```python
from build123d import *

# Parameters (mm, degrees)
SKETCH1_W           = 60
SKETCH1_H           = 15
SKETCH1_R           = 1
BOSS_EXTRUDE1_DEPTH = 4
FILLET1_RADIUS      = 7.5
FILLET1_LENGTH      = 4
FILLET2_RADIUS      = 7.5
FILLET2_LENGTH      = 4
CUT_EXTRUDE1_DEPTH  = 2
SKETCH4_R           = 3.5
CUT_EXTRUDE2_DEPTH  = 6
CUT_EXTRUDE3_DEPTH  = 2
SKETCH6_R           = 3.5
CUT_EXTRUDE4_DEPTH  = 6


with BuildPart() as part:
    # Sketch1 → Boss-Extrude1 (new body)
    with BuildSketch(Plane.XY):
        with Locations((-25, 9.186746988)):
            Rectangle(SKETCH1_W, SKETCH1_H)
        with Locations((-50, 9.186746988)):
            Circle(SKETCH1_R, mode=Mode.SUBTRACT)
        with Locations((0, 9.186746988)):
            Circle(SKETCH1_R, mode=Mode.SUBTRACT)
    extrude(amount=BOSS_EXTRUDE1_DEPTH)

    # Fillet1: full round fillet: the end face becomes a half cylinder, R = half its width
    fillet1_face = Plane((5, 9.186746988, 2), x_dir=(0, 0, -1), z_dir=(1, 0, 0))  # on the end face: x along it, z out of the body
    fillet1_slab = fillet1_face.offset(-FILLET1_RADIUS / 2) * Box(FILLET1_LENGTH, 2 * FILLET1_RADIUS, FILLET1_RADIUS, mode=Mode.PRIVATE)  # the body's end, R deep
    fillet1_round = Plane((-2.5, 9.186746988, 2), x_dir=(1, 0, 0), z_dir=(0, 0, -1)) * Cylinder(FILLET1_RADIUS, FILLET1_LENGTH, mode=Mode.PRIVATE)  # its axis R under the face
    add(fillet1_slab - fillet1_round, mode=Mode.SUBTRACT)

    # Fillet2: full round fillet: the end face becomes a half cylinder, R = half its width
    fillet2_face = Plane((-55, 9.186746988, 2), x_dir=(0, 0, 1), z_dir=(-1, 0, 0))  # on the end face: x along it, z out of the body
    fillet2_slab = fillet2_face.offset(-FILLET2_RADIUS / 2) * Box(FILLET2_LENGTH, 2 * FILLET2_RADIUS, FILLET2_RADIUS, mode=Mode.PRIVATE)  # the body's end, R deep
    fillet2_round = Plane((-47.5, 9.186746988, 2), x_dir=(-1, 0, 0), z_dir=(0, 0, 1)) * Cylinder(FILLET2_RADIUS, FILLET2_LENGTH, mode=Mode.PRIVATE)  # its axis R under the face
    add(fillet2_slab - fillet2_round, mode=Mode.SUBTRACT)

    # Sketch3 → Cut-Extrude1 (cut)
    with BuildSketch(Plane(origin=(0, 0, 0), x_dir=(-1, 0, 0), z_dir=(0, 0, -1))):
        with BuildLine():
            Line((14.214285714, 11.17523426), (0.375, 12.666599715))
            ThreePointArc((0.375, 12.666599715), (-3.5, 9.186746988), (0.375, 5.706894261))
            Line((0.375, 5.706894261), (14.214285714, 7.198259716))
            ThreePointArc((14.214285714, 7.198259716), (16, 9.186746988), (14.214285714, 11.17523426))
        make_face()
    extrude(amount=-CUT_EXTRUDE1_DEPTH, mode=Mode.SUBTRACT)

    # Sketch4 → Cut-Extrude2 (cut)
    with BuildSketch(Plane(origin=(0, 0, 2), x_dir=(-1, 0, 0), z_dir=(0, 0, -1))):
        with Locations(Location((0, 9.186746988, 0), (0, 0, 276.150639828))):
            Circle(SKETCH4_R)
    extrude(amount=-CUT_EXTRUDE2_DEPTH, mode=Mode.SUBTRACT)

    # Sketch5 → Cut-Extrude3 (cut)
    with BuildSketch(Plane(origin=(0, 0, 0), x_dir=(-1, 0, 0), z_dir=(0, 0, -1))):
        with BuildLine():
            Line((49.625, 12.666599715), (35.785714286, 11.17523426))
            ThreePointArc((35.785714286, 11.17523426), (34, 9.186746988), (35.785714286, 7.198259716))
            Line((35.785714286, 7.198259716), (49.625, 5.706894261))
            ThreePointArc((49.625, 5.706894261), (53.5, 9.186746988), (49.625, 12.666599715))
        make_face()
    extrude(amount=-CUT_EXTRUDE3_DEPTH, mode=Mode.SUBTRACT)

    # Sketch6 → Cut-Extrude4 (cut)
    with BuildSketch(Plane(origin=(0, 0, 0), x_dir=(-1, 0, 0), z_dir=(0, 0, -1))):
        with Locations(Location((50, 9.186746988, 0), (0, 0, 96.150639828))):
            Circle(SKETCH6_R)
    extrude(amount=-CUT_EXTRUDE4_DEPTH, mode=Mode.SUBTRACT)


solid = part.part
```
Source: CAD feature listing. Evaluate the final solid. Frame: model axes, mm. A direction names the side the tool comes from. Round coordinates to 2 decimals unless told otherwise and drop trailing zeros. Write each loop counter-clockwise with the first axis right and the second up, starting at its lowest first coordinate (ties: lowest second). Pieces come first, ordered by that corner, then holes. Notation, with made-up numbers: M -29.5,1 L -14.5,1 A31 ccw -14.5,32 Z; hole C -38,-37 d7. An arc over 180 degrees is marked long. Answer as a JSON object with one key per item and string values. Group by question number.
(1) Section query C-C on y = 9.25. Output: boundary loops of the cut face in (x, z), then the cut area to 3 significant figures.
(2) Reachability of faces 1 (the flat face through (-25, 9, 4)), 2 (the flat face through (-42.608, 6.463, 0.986)) from +Z, -Z, +X, -X, +Y, -Y: full face, straight path, thin tool, end or side. Return the list, or none.
(3) First-contact query: pin 1 (2 mm diameter, centred on x = -39.5, y = 9, fed in from -Z); pin 2 (7.5 mm diameter, centred on x = -7.5, y = 8.5, fed in from -Z). Flat tips, straight axial feed; report the tip coordinate or a pass-through.
(4) Ray query, line 1 (X direction, y = 11, z = 1.1); line 2 (X direction, y = 6.25, z = 2.4); line 3 (Z direction, x = -41, y = 11.5). Return the intervals inside material, ascending. Write a range as [from, to].
(5) Mould query, pull axis Y, two halves, no side actions, for faces 3 (the flat face through (-7.198, 6.442, 0.986)), 4 (the cylindrical face through (-55, 9.35, 2.03)), 5 (the flat face through (-25, 1.687, 2)). Classes: +Y half, -Y half, draft (parallel to the pull), parting line (faces both ways), or undercut.
(6) Section query D-D on z = 3.05. Output: boundary loops of the cut face in (x, y) (3 decimals), then the cut area to 3 significant figures.
(7) Section query A-A on x = -48.5. Output: boundary loops of the cut face in (y, z).
(8) Section query B-B on z = 0.85. Output: boundary loops of the cut face in (x, y) (3 decimals), then the cut area to 3 significant figures.
Computed values:
{
 "1": {"outline": "M -55,0 L -53.5,0 L -53.5,4 L -55,4 Z; M -46.5,2 L -34,2 L -34,0 L -16,0 L -16,2 L -3.5,2 L -3.5,4 L -46.5,4 Z; M 3.5,0 L 5,0 L 5,4 L 3.5,4 Z", "area": "134 mm^2"},
 "2": {"face 1": "+Z, +X, -X, +Y, -Y", "face 2": "-Z"},
 "3": {"pin 1": "z = 2", "pin 2": "z = 0"},
 "4": {"line 1": "[-54.78, -52.99], [-35.16, -14.84], [2.99, 4.78]", "line 2": "[-54.4, -51.9], [-48.1, -1.9], [1.9, 4.4]", "line 3": "[2, 4]"},
 "5": {"face 3": "undercut", "face 4": "parting line", "face 5": "-Y half"},
 "6": {"outline": "M -47.5,1.687 L -2.5,1.687 A7.5 ccw -2.5,16.687 L -47.5,16.687 A7.5 ccw Z; hole C -50,9.187 d7; hole C 0,9.187 d7", "area": "775 mm^2"},
 "7": {"outline": "M 1.75,0 L 5.83,0 L 5.83,2 L 6.02,2 L 6.02,4 L 1.75,4 Z; M 12.35,2 L 12.55,2 L 12.55,0 L 16.62,0 L 16.62,4 L 12.35,4 Z"},
 "8": {"outline": "M -47.5,1.687 L -2.5,1.687 A7.5 ccw -2.5,16.687 L -47.5,16.687 A7.5 ccw Z; hole M -49.625,5.707 L -35.786,7.198 A2 ccw -35.786,11.175 L -49.625,12.667 A3.5 ccw long Z; hole M -14.214,7.198 L -0.375,5.707 A3.5 ccw long -0.375,12.667 L -14.214,11.175 A2 ccw Z", "area": "646 mm^2"}
}
